For this review, take the finished solid that the model builds, in its own axes (mm). Face numbers are marked on the shaded views. A direction names the side the tool comes from. Round coordinates to 2 decimals unless told otherwise and drop trailing zeros. Order: outer loops, then holes, each group sorted by start corner. A loop starts at its lowest first (then second) coordinate and runs counter-clockwise, first axis right, second up. Notation, with made-up numbers: M 39.5,-31.5 L 84.5,-31.5 A16 ccw 84.5,-14.5 Z; hole C 82.25,-23.75 d2. An arc over 180 degrees is marked long. Write item = value, one per line. Start each with the question number.
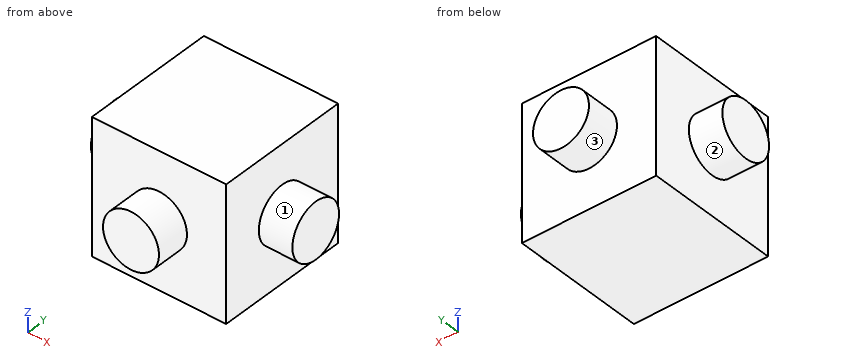
from build123d import *

# Parameters (mm, degrees)
SKETCH_1_W           = 12
SKETCH_1_H           = 12
EXTRUDE_1_DEPTH      = 12
EXTRUDE_2_DEPTH      = 3
EXTRUDE_2_DEPTH_BACK = 15
SKETCH_2_R           = 2.5
EXTRUDE_3_DEPTH      = 3
EXTRUDE_3_DEPTH_BACK = 15
SKETCH_3_R           = 2.5


with BuildPart() as part:
    # 草图1 → 凸台-拉伸1 (new body)
    with BuildSketch(Plane(origin=(0, 0, 0), x_dir=(1, 0, 0), z_dir=(0, 1, 0))):
        Rectangle(SKETCH_1_W, SKETCH_1_H)
    extrude(amount=EXTRUDE_1_DEPTH)

    # 草图2 → 凸台-拉伸2 (add, two sides: drawn at the far end of the back side and taken through both)
    with BuildSketch(Plane(origin=(0, 12, 0), x_dir=(1, 0, 0), z_dir=(0, 1, 0)).offset(-EXTRUDE_2_DEPTH_BACK)):
        with Locations(Location((0, 0, 0), (0, 0, 270))):
            Circle(SKETCH_2_R)
    extrude(amount=EXTRUDE_2_DEPTH + EXTRUDE_2_DEPTH_BACK)

    # 草图3 → 凸台-拉伸3 (add, two sides: drawn at the far end of the back side and taken through both)
    with BuildSketch(Plane(origin=(6, 0, 0), x_dir=(0, 0, -1), z_dir=(1, 0, 0)).offset(-EXTRUDE_3_DEPTH_BACK)):
        with Locations((0, 6)):
            Circle(SKETCH_3_R)
    extrude(amount=EXTRUDE_3_DEPTH + EXTRUDE_3_DEPTH_BACK)


solid = part.part
(1) We need section B-B, the plane z = 0. Write out the cut boundary in (x, y).
(2) For line 1 along Y through (x, z) = (-5, 5); line 2 along X through (y, z) = (0.5, 1.5); line 3 along Y through (x, z) = (7.5, -2.25), list the stretches that pass through material, from the lowest coordinate up.
(3) We need section C-C, the plane y = 6. Write out the cut boundary in (x, z), then the cut area to 3 significant figures.
(4) For the marked faces 1, 2 and 3, list the 3-axis set-ups (+Z, -Z, +X, -X, +Y, -Y) from which the entire face can be reached by the end or side of a thin tool; tool diameter is ignored.
(5) We need section A-A, the plane x = 0. Write out the cut boundary in (y, z).
(6) Insertion check: pin 1 (5 mm diameter, centred on x = -6.5, z = 1, fed in from -Y); pin 2 (1.5 mm diameter, centred on x = 4, z = -3, fed in from +Y). Each pin has a flat end and moves straight along its axis. Give the tip position at first contact, or say it passes through.
(7) We need section D-D, the plane x = -5.75. Write out the cut boundary in (y, z), then the cut area to 3 significant figures.
Values:
q1.outline = M -9,3.5 L -6,3.5 L -6,0 L -2.5,0 L -2.5,-3 L 2.5,-3 L 2.5,0 L 6,0 L 6,3.5 L 9,3.5 L 9,8.5 L 6,8.5 L 6,12 L 2.5,12 L 2.5,15 L -2.5,15 L -2.5,12 L -6,12 L -6,8.5 L -9,8.5 Z
q2.line_1 = 0 to 12
q2.line_2 = -6 to 6
q2.line_3 = 4.91 to 7.09
q3.outline = M -9,-2.5 L -6,-2.5 L -6,-6 L 6,-6 L 6,-2.5 L 9,-2.5 L 9,2.5 L 6,2.5 L 6,6 L -6,6 L -6,2.5 L -9,2.5 Z
q3.area = 174 mm²
q4.face_1 = +X
q4.face_2 = -X
q4.face_3 = +Y
q5.outline = M -3,-2.5 L 0,-2.5 L 0,-6 L 12,-6 L 12,-2.5 L 15,-2.5 L 15,2.5 L 12,2.5 L 12,6 L 0,6 L 0,2.5 L -3,2.5 Z
q6.pin_1 = 0
q6.pin_2 = 12
q7.outline = M 0,-6 L 12,-6 L 12,6 L 0,6 Z
q7.area = 144 mm²
